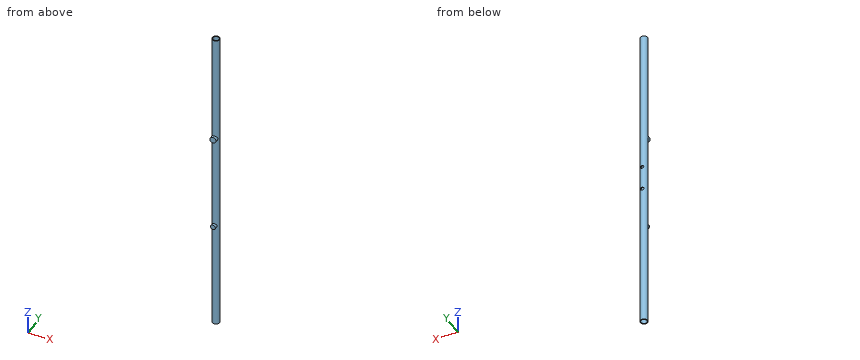
```python
from build123d import *

# Parameters (mm, degrees)
F0_R     = 15
F0_R_2   = 12
F1_DEPTH = 1300
F2_R     = 6.699754
F2_R_2   = 6.23735
F3_DEPTH = 25
F4_R     = 10
F4_R_2   = 12.5
F5_DEPTH = 25


with BuildPart() as f1:
    # F0 (on Top) → F1 (new body)
    with BuildSketch(Plane.XY):
        Circle(F0_R)
        Circle(F0_R_2, mode=Mode.SUBTRACT)
    extrude(amount=F1_DEPTH)

    # F2 (on Front) → F3 (cut)
    with BuildSketch(Plane.XZ):
        with Locations((0, 600)):
            Circle(F2_R)
        with Locations((0, 700)):
            Circle(F2_R_2)
    extrude(amount=-F3_DEPTH, mode=Mode.SUBTRACT)

    # F4 (on Front) → F5 (join)
    with BuildSketch(Plane.XZ):
        with Locations((0, 450)):
            Circle(F4_R)
        with Locations((0, 850)):
            Circle(F4_R_2)
    extrude(amount=F5_DEPTH)


solid = f1.part
```
Can you work these out from the model? Positions are in its coordinate system, mm. Round coordinates to 2 decimals unless told otherwise and drop trailing zeros. Loops run counter-clockwise (first coordinate to the right, second up) from the corner with the lowest first, then second, coordinate; pieces in that order, holes last. Notation, with made-up numbers: (-36, 26.5) -> (6, 26.5) arc R26 cw to (6, 51.5) -> close; hole circle Ø1 at (11, 23). An arc over 180 degrees is marked (long way). One line per item, written item: value. Start each with the question number.
1. If I drill on probe 1 along Z at (x, y) = (0, 14.05); probe 2 along X at (y, z) = (1.5, 1089); probe 3 along X at (y, z) = (11.4, 600), over which ranges is the centre line in solid material (lowest first)?
2. If we section it at A-A, the plane z = 376.5: Write out the boundary of the cut face in (x, y).
3. For pin 1 (11 mm diameter, centred on x = 0, z = 700, fed in from +Y); pin 2 (10.5 mm diameter, centred on x = 0, z = 600, fed in from +Y); pin 3 (2 mm diameter, centred on y = 9, z = 971, fed in from -X), each with a flat end and sliding along its axis, tell me the tip position at first contact or that it passes through.
Calculated:
1. probe 1: z = 0 to 593.3, 606.7 to 693.76, 706.24 to 1300
1. probe 2: x = -14.92 to -11.91, 11.91 to 14.92
1. probe 3: x = -9.75 to -6.7, 6.7 to 9.75
2. outline: circle Ø30 at (0, 0); hole circle Ø24 at (0, 0)
3. pin 1: stops at y = -10.67
3. pin 2: stops at y = -10.79
3. pin 3: stops at x = -12.69
